CAD build for the part. Positions are in the model's coordinates, mm. A direction names the side the tool comes from. Round coordinates to 2 decimals unless told otherwise and drop trailing zeros. Loops run counter-clockwise (first coordinate to the right, second up) from the corner with the lowest first, then second, coordinate; pieces in that order, holes last. Notation, with made-up numbers: M 78,51.5 L 132,51.5 A7 cw 132,57.5 Z; hole C 3.5,58 d7. An arc over 180 degrees is marked long. Use a Markdown table: item, result. Add a question column.
(1) Flat gauge pins, fed straight in: P1, Ø1.6, axis at x = 24, z = -36.5, coming from the -Y side; P2, Ø3, axis at x = 40, z = -8.5, coming from the +Y side; P3, Ø12, axis at x = 21.5, y = 15.5, coming from the -Z side; P4, Ø4, axis at x = 7.5, z = -30, coming from the +Y side. Where does each tip first touch, or does it go through?
(2) Band-saw the part on A-A, the plane x = 25. Write the cut outline in (y, z).
(3) Two-plate mould, pull along Z, no slides. Class faces 1 (the face through (50, 2, -17)), 2 (the face through (45.879, 4.507, -33.685)), 3 (the face through (25, 2, -40)), 4 (the face through (25, 8, 0)): released by +Z, released by -Z, zero draft, split by the parting line, or undercut.
(4) Which spindle directions (+Z, -Z, +X, -X, +Y, -Y) get a long thin tool onto all of the face, cutting with end or side? Do faces 5 (the face through (37, 9, -19)), 6 (the face through (9, 4.51, -5.23)), 7 (the face through (13, 9, -19)), 8 (the face through (25, 0, -20)), 9 (the face through (25.264, 3.383, -22.847)). Say none if no direction does.
(5) Band-saw the part on B-B, the plane x = 46. Write the cut outline in (y, z).
(6) Wall check: L1, parallel to X at y = 19.75, z = -10.5; L2, parallel to Z at x = 33, y = 19.5; L3, parallel to Z at x = 9, y = 2. Give the ranges that are in metal, low to high.
from build123d import *

# Parameters (mm, degrees)
BOSS_EXTRUDE1_DEPTH           = 5
SKETCH2_R                     = 12
SKETCH2_R_2                   = 5.4
SKETCH2_R_3                   = 1.55
BOSS_EXTRUDE2_DEPTH           = 12.25
BOSS_EXTRUDE3_DEPTH           = 4.5
CHAMFER1_SIZE                 = 2
BOSS_EXTRUDE4_DEPTH           = 24
SKETCH5_R                     = 5.4
SKETCH5_R_2                   = 1.55
CUT_EXTRUDE1_DEPTH            = 70.639531877
CUT_EXTRUDE2_START            = -27.75
SKETCH6_R                     = 12
CUT_EXTRUDE2_DEPTH            = 27.75
FILLET1_R                     = 5.5
BOSS_EXTRUDE5_DEPTH           = 1
BOSS_EXTRUDE5_DRAFT           = 45
SKETCH7_W                     = 50
SKETCH7_H                     = 9
BOSS_EXTRUDE5_PROFILE_2_DEPTH = 1
BOSS_EXTRUDE5_PROFILE_2_DRAFT = 45
SKETCH8_R                     = 2.5
CUT_EXTRUDE3_DEPTH            = 71.038734997
SKETCH9_R                     = 5
CUT_EXTRUDE4_DEPTH            = 1


with BuildPart() as part:
    # Sketch1 → Boss-Extrude1 (new body)
    with BuildSketch(Plane(origin=(0, 0, 0), x_dir=(1, 0, 0), z_dir=(0, 1, 0))):
        with BuildLine():
            Line((0, 2), (2, 0))
            Line((2, 0), (48, 0))
            Line((48, 0), (50, 2))
            Line((50, 2), (50, 32.5))
            ThreePointArc((50, 32.5), (47.803300859, 37.803300859), (42.5, 40))
            Line((42.5, 40), (7.5, 40))
            ThreePointArc((7.5, 40), (2.196699141, 37.803300859), (0, 32.5))
            Line((0, 32.5), (0, 2))
        make_face()
    extrude(amount=BOSS_EXTRUDE1_DEPTH)

    # Sketch2 → Boss-Extrude2 (add)
    with BuildSketch(Plane.XY):
        with Locations((25, 15.38)):
            Circle(SKETCH2_R)
        with Locations((25, 15.38)):
            Circle(SKETCH2_R_2, mode=Mode.SUBTRACT)
        with Locations((19.33, 21.05)):
            Circle(SKETCH2_R_3, mode=Mode.SUBTRACT)
        with Locations(Location((30.67, 21.05, 0), (0, 0, 180))):
            Circle(SKETCH2_R_3, mode=Mode.SUBTRACT)
        with Locations((30.67, 9.71)):
            Circle(SKETCH2_R_3, mode=Mode.SUBTRACT)
        with Locations(Location((19.33, 9.71, 0), (0, 0, 180))):
            Circle(SKETCH2_R_3, mode=Mode.SUBTRACT)
    extrude(amount=-BOSS_EXTRUDE2_DEPTH)

    # Sketch3 → Boss-Extrude3 (add)
    with BuildSketch(Plane.XY):
        with BuildLine():
            Line((13, 15.38), (0, 5))
            Line((0, 5), (18.978737674, 5))
            ThreePointArc((18.978737674, 5), (14.601559061, 9.390640598), (13, 15.38))
        make_face()
        with BuildLine():
            Line((50, 5), (31.021262326, 5))
            ThreePointArc((31.021262326, 5), (35.398440939, 9.390640598), (37, 15.38))
            Line((37, 15.38), (50, 5))
        make_face()
    extrude(amount=-BOSS_EXTRUDE3_DEPTH)

    # Chamfer1
    # the kernel refuses this chamfer: 2 mm, written as the material it takes off along each edge
    with BuildSketch(Plane(origin=(32.980691337, 18.589263379, 0), x_dir=(-0.6237257907466237, -0.7811594681797787, 0.027495876610586348), z_dir=(0.7814549230707756, -0.6239617001134351, 0))) as chamfer1_piece_1_section:
        Polygon((CHAMFER1_SIZE * 0.999621916911, CHAMFER1_SIZE * 0.0274958766106), (-CHAMFER1_SIZE * 0.0274958766106, CHAMFER1_SIZE * 0.999621916911), (0, 0), align=None)
    chamfer1_piece_1 = extrude(amount=26.922368399, mode=Mode.PRIVATE)
    chamfer1_piece_1 = chamfer1_piece_1 - Plane(origin=(25, 15.38, -0.663889937), x_dir=(1, 0, 0), z_dir=(0, 0, 1)) * Cylinder(12, 62, mode=Mode.PRIVATE)
    add(chamfer1_piece_1, mode=Mode.SUBTRACT)
    with BuildSketch(Plane(origin=(17.019308663, 18.589263379, 0), x_dir=(-0.017156373916051248, 0.02148678814149, -0.9996219169112968), z_dir=(-0.7814549230707758, -0.6239617001134349, 0))) as chamfer1_piece_2_section:
        Polygon((CHAMFER1_SIZE * 0.999621916911, CHAMFER1_SIZE * 0.0274958766106), (-CHAMFER1_SIZE * 0.0274958766106, CHAMFER1_SIZE * 0.999621916911), (0, 0), align=None)
    chamfer1_piece_2 = extrude(amount=26.922368399, mode=Mode.PRIVATE)
    chamfer1_piece_2 = chamfer1_piece_2 - Plane(origin=(25, 15.38, -0.663889938), x_dir=(1, 0, 0), z_dir=(0, 0, 1)) * Cylinder(12, 62, mode=Mode.PRIVATE)
    add(chamfer1_piece_2, mode=Mode.SUBTRACT)

    # Sketch4 → Boss-Extrude4 (add)
    with BuildSketch(Plane.ZY.offset(-13)):
        Polygon((-40, 5), (-4.5, 5), (-4.5, 15.38), (-12.25, 15.38), align=None)
    extrude(amount=-BOSS_EXTRUDE4_DEPTH)

    # Sketch5 → Cut-Extrude1 (cut, through all)
    with BuildSketch(Plane.XY):
        with Locations((25, 15.38)):
            Circle(SKETCH5_R)
        with Locations((30.67, 9.71)):
            Circle(SKETCH5_R_2)
        with Locations(Location((19.33, 9.71, 0), (0, 0, 90))):
            Circle(SKETCH5_R_2)
    extrude(amount=-CUT_EXTRUDE1_DEPTH, mode=Mode.SUBTRACT)

    # Sketch6 → Cut-Extrude2 (cut)
    with BuildSketch(Plane(origin=(0, 0, -40), x_dir=(-1, 0, 0), z_dir=(0, 0, -1)).offset(CUT_EXTRUDE2_START)):
        with Locations((-25, 15.38)):
            Circle(SKETCH6_R)
    extrude(amount=CUT_EXTRUDE2_DEPTH, mode=Mode.SUBTRACT)

    # Fillet1
    # the kernel refuses this fillet: 5.5 mm, written as the material it adds along each edge
    with BuildSketch(Plane(origin=(13, 5, -4.5), x_dir=(0, 0, -1), z_dir=(0, 1, 0))) as fillet1_piece_1_section:
        with BuildLine():
            CenterArc((FILLET1_R, FILLET1_R), FILLET1_R, 180, 90)
            Line((0, FILLET1_R), (0, 0))
            Line((0, 0), (FILLET1_R, 0))
        make_face()
    fillet1_piece_1 = extrude(amount=24.13, mode=Mode.PRIVATE)
    fillet1_piece_1 = split(fillet1_piece_1, bisect_by=Plane(origin=(9.562905038, 12.635611869, -5.815830527), z_dir=(0.6239617001134349, -0.7814549230707758, 0)), keep=Keep.TOP, mode=Mode.PRIVATE)
    add(fillet1_piece_1)
    with BuildSketch(Plane(origin=(37, 5, -4.5), x_dir=(1, 0, 0), z_dir=(0, 1, 0))) as fillet1_piece_2_section:
        with BuildLine():
            CenterArc((FILLET1_R, FILLET1_R), FILLET1_R, 180, 90)
            Line((0, FILLET1_R), (0, 0))
            Line((0, 0), (FILLET1_R, 0))
        make_face()
    fillet1_piece_2 = extrude(amount=24.13, mode=Mode.PRIVATE)
    fillet1_piece_2 = split(fillet1_piece_2, bisect_by=Plane(origin=(40.437094962, 12.635611869, -5.815830527), z_dir=(-0.6239617001134351, -0.7814549230707756, 0)), keep=Keep.TOP, mode=Mode.PRIVATE)
    add(fillet1_piece_2)


with BuildPart() as boss_extrude5_tool:
    # Sketch7 → Boss-Extrude5 (with draft: the straight prism first)
    with BuildSketch(Plane.XZ):
        with BuildLine():
            Line((0, -25.5), (0, -32.5))
            ThreePointArc((0, -32.5), (0.068206101, -33.509177609), (0.271583853, -34.5))
            Line((0.271583853, -34.5), (49.728416147, -34.5))
            ThreePointArc((49.728416147, -34.5), (49.931793899, -33.509177609), (50, -32.5))
            Line((50, -32.5), (50, -25.5))
            Line((50, -25.5), (0, -25.5))
        make_face()
    extrude(amount=BOSS_EXTRUDE5_DEPTH)
    # Boss-Extrude5: the draft: its side faces are tilted about the plane it starts from
    boss_extrude5_sides = [boss_extrude5_tool.faces().sort_by_distance(p)[0] for p in [
        (0, -0.5, -29),
        (0.068206101, -0.5, -33.509177609),
        (25, -0.5, -34.5),
        (49.931793899, -0.5, -33.509177609),
        (50, -0.5, -29),
        (25, -0.5, -25.5),
    ]]
    draft(boss_extrude5_sides, Plane.XZ, BOSS_EXTRUDE5_DRAFT)


with BuildPart() as part_1:
    add(part.part)

    # Boss-Extrude5: add boss_extrude5_tool
    add(boss_extrude5_tool.part)


with BuildPart() as boss_extrude5_profile_2_tool:
    # Sketch7 → Boss-Extrude5 profile 2 (with draft: the straight prism first)
    with BuildSketch(Plane.XZ):
        with Locations((25, -10)):
            Rectangle(SKETCH7_W, SKETCH7_H)
    extrude(amount=BOSS_EXTRUDE5_PROFILE_2_DEPTH)
    # Boss-Extrude5 profile 2: the draft: its side faces are tilted about the plane it starts from
    boss_extrude5_profile_2_sides = [boss_extrude5_profile_2_tool.faces().sort_by_distance(p)[0] for p in [
        (0, -0.5, -10),
        (25, -0.5, -14.5),
        (50, -0.5, -10),
        (25, -0.5, -5.5),
    ]]
    draft(boss_extrude5_profile_2_sides, Plane.XZ, BOSS_EXTRUDE5_PROFILE_2_DRAFT)


with BuildPart() as part_2:
    add(part_1.part)

    # Boss-Extrude5 profile 2: add boss_extrude5_profile_2_tool
    add(boss_extrude5_profile_2_tool.part)

    # Sketch8 → Cut-Extrude3 (cut, through all)
    with BuildSketch(Plane.XZ.offset(1)):
        with Locations(Location((7.5, -30, 0), (0, 0, 270))):
            Circle(SKETCH8_R)
        with Locations(Location((42.5, -30, 0), (0, 0, 270))):
            Circle(SKETCH8_R)
        with Locations(Location((42.5, -10, 0), (0, 0, 270))):
            Circle(SKETCH8_R)
        with Locations(Location((7.5, -10, 0), (0, 0, 270))):
            Circle(SKETCH8_R)
    extrude(amount=-CUT_EXTRUDE3_DEPTH, mode=Mode.SUBTRACT)

    # Sketch9 → Cut-Extrude4 (cut)
    with BuildSketch(Plane(origin=(0, 5, 0), x_dir=(1, 0, 0), z_dir=(0, 1, 0))):
        with Locations(Location((7.5, 30, 0), (0, 0, 270))):
            Circle(SKETCH9_R)
        with Locations(Location((7.5, 10, 0), (0, 0, 270))):
            Circle(SKETCH9_R)
        with Locations(Location((42.5, 30, 0), (0, 0, 270))):
            Circle(SKETCH9_R)
        with Locations(Location((42.5, 10, 0), (0, 0, 270))):
            Circle(SKETCH9_R)
    extrude(amount=-CUT_EXTRUDE4_DEPTH, mode=Mode.SUBTRACT)


solid = part_2.part
Return value:
| question | item | result |
|---|---|---|
| 1 | P1 | y = 0 |
| 1 | P2 | y = 4 |
| 1 | P3 | z = -12.25 |
| 1 | P4 | through |
| 2 | outline | M -1,-33.5 L 0,-34.5 L 0,-40 L 3.38,-40 L 3.38,-12.25 L 9.98,-12.25 L 9.98,0 L 0,0 L 0,-5.5 L -1,-6.5 L -1,-13.5 L 0,-14.5 L 0,-25.5 L -1,-26.5 Z; M 20.78,-12.25 L 27.38,-12.25 L 27.38,0 L 20.78,0 Z |
| 3 | face 1 | zero draft |
| 3 | face 2 | undercut |
| 3 | face 3 | released by -Z |
| 3 | face 4 | released by +Z |
| 4 | face 5 | -Z, +X, +Y |
| 4 | face 6 | +Y |
| 4 | face 7 | -Z, -X, +Y |
| 4 | face 8 | +X, -X, -Y |
| 4 | face 9 | -Z, +Y |
| 5 | outline | M -1,-33.5 L 0,-34.5 L 0,-39.13 L 5,-39.13 L 5,-33.57 L 4,-33.57 L 4,-26.43 L 5,-26.43 L 5,-13.57 L 4,-13.57 L 4,-6.43 L 5,-6.43 L 5,-4.5 L 8.19,-4.5 L 8.19,-2 L 5.63,0 L 0,0 L 0,-5.5 L -1,-6.5 L -1,-13.5 L 0,-14.5 L 0,-25.5 L -1,-26.5 Z |
| 6 | L1 | 13.82 to 18.49, 20.17 to 21.83, 28.17 to 29.83, 31.51 to 36.18 |
| 6 | L2 | -12.25 to 0 |
| 6 | L3 | -40 to -32, -28 to -12, -8 to 0 |
